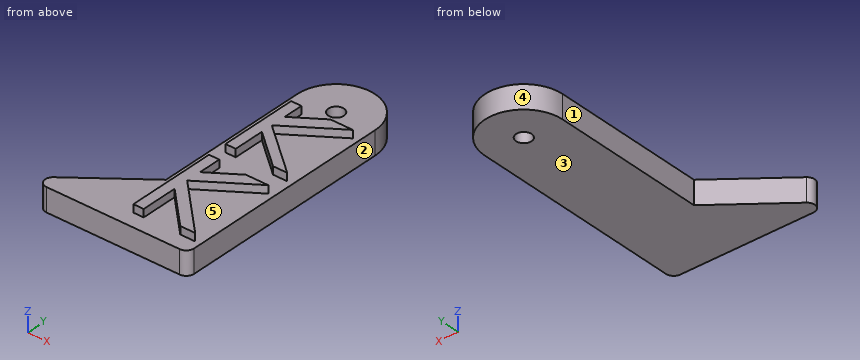
```python
from build123d import *

# Parameters (mm, degrees)
SKETCH_1_R      = 1
EXTRUDE_1_DEPTH = 3
EXTRUDE_2_DEPTH = 3
FILLET_2_R      = 1
FILLET_3_R      = 1
EXTRUDE_3_DEPTH = 1


with BuildPart() as part:
    # 草图1 → 凸台-拉伸1 (new body)
    with BuildSketch(Plane.XY):
        with BuildLine():
            Line((-5, 0), (-5, -20))
            Line((-5, -20), (5, -20))
            Line((5, -20), (5, 0))
            ThreePointArc((5, 0), (0, 5), (-5, 0))
        make_face()
        Circle(SKETCH_1_R, mode=Mode.SUBTRACT)
    extrude(amount=EXTRUDE_1_DEPTH)

    # 草图2 → 凸台-拉伸2 (add)
    with BuildSketch(Plane.XY.offset(3)):
        Polygon((5, -20), (-5, -20), (-16.053330201, -28.571505672), (5, -28.571505672), align=None)
    extrude(amount=-EXTRUDE_2_DEPTH)

    # 圆角2
    fillet_2_edges = [part.edges().sort_by_distance(p)[0] for p in [
        (-16.053330201, -28.571505672, 1.5),
    ]]
    fillet(fillet_2_edges, radius=FILLET_2_R)

    # 圆角3
    fillet_3_edges = [part.edges().sort_by_distance(p)[0] for p in [
        (5, -28.571505672, 1.5),
    ]]
    fillet(fillet_3_edges, radius=FILLET_3_R)

    # 草图3 → 凸台-拉伸3 (add)
    with BuildSketch(Plane.XY.offset(3)):
        Polygon((-3.674988176, -2.510402489), (-3.674988176, -12.516814932), (-2.349938126, -12.516814932), (-2.349938126, -8.541664784), (2.447656881, -12.516814932), (4.275312121, -12.516814932), (-2.349938126, -7.02732187), (4.275312121, -2.510402489), (1.392652218, -2.510402489), (-2.349938126, -5.062001029), (-2.349938126, -2.510402489), align=None)
        Polygon((-3.674988176, -15.023538628), (-3.674988176, -26.544068904), (-2.349938126, -26.544068904), (-2.349938126, -21.837856659), (2.356274118, -26.544068904), (4.275312121, -26.544068904), (-2.349938126, -19.918818657), (4.275312121, -15.401899276), (1.392652218, -15.401899276), (-2.349938126, -17.953497816), (-2.349938126, -15.023538628), align=None)
    extrude(amount=EXTRUDE_3_DEPTH)


solid = part.part
```
Source: CAD feature listing. Evaluate the final solid. Frame: model axes, mm. Face numbers are marked on the shaded views. A direction names the side the tool comes from. Coordinates: 2 decimals unless noted, no trailing zeros. Write each loop counter-clockwise with the first axis right and the second up, starting at its lowest first coordinate (ties: lowest second). Pieces come first, ordered by that corner, then holes. Notation, with made-up numbers: (-35, 19.5) -> (-28, 19.5) arc R27 ccw to (-28, 48.5) -> close; hole circle Ø4 at (-31, 24.25). An arc over 180 degrees is marked (long way). Return JSON: item names as keys, results as strings. Group by question number.
1) Section query D-D, the plane x = -10.25. Return loops of the section in (y, z).
2) Section query B-B, the plane x = 0. Return loops of the section in (y, z).
3) Mould query, pull axis Y, two halves, no side actions, for the marked faces 3, 4 and 5. Classes: +Y half, -Y half, draft (parallel to the pull), parting line (faces both ways), or undercut.
4) Contact query for flat-ended pins moving along their axis: P1, Ø0.5, axis at y = -9.5, z = 3.5, coming from the +X side; P2, Ø1.8, axis at x = 0, y = 0, coming from the +Z side; P3, Ø1, axis at y = -24.5, z = 2, coming from the -X side; P4, Ø0.5, axis at y = -9.5, z = 3.5, coming from the -X side (3 decimals). Output: stop coordinate, or through.
5) Ray query, line 1 along Y through (x, z) = (0, 2.35); line 2 along Y through (x, z) = (-2.5, 3.4); line 3 along X through (y, z) = (-9.5, 1.55). Return the intervals inside material, ascending.
6) Set-up query: the marked faces 1 and 2. Return all of +Z, -Z, +X, -X, +Y, -Y with unobstructed straight access to the full face (end or side cutting, diameter ignored); none if empty.
7) Section query A-A, the plane z = 0.55. Return loops of the section in (x, y).
8) Section query C-C, the plane y = -4. Return loops of the section in (x, z), plus the area to 3 significant figures.
From the geometry:
{
 "1": {"outline": "(-28.57, 0) -> (-24.07, 0) -> (-24.07, 3) -> (-28.57, 3) -> close"},
 "2": {"outline": "(-28.57, 0) -> (-1, 0) -> (-1, 3) -> (-3.46, 3) -> (-3.46, 4) -> (-5.43, 4) -> (-5.43, 3) -> (-8.97, 3) -> (-8.97, 4) -> (-10.49, 4) -> (-10.49, 3) -> (-16.35, 3) -> (-16.35, 4) -> (-18.32, 4) -> (-18.32, 3) -> (-22.27, 3) -> (-22.27, 4) -> (-24.19, 4) -> (-24.19, 3) -> (-28.57, 3) -> close; (1, 0) -> (5, 0) -> (5, 3) -> (1, 3) -> close"},
 "3": {"face 3": "draft", "face 4": "+Y half", "face 5": "undercut"},
 "4": {"P1": "x = 0.94", "P2": "through", "P3": "x = -11.45", "P4": "x = -3.675"},
 "5": {"line 1": "-28.57 to -1, 1 to 5", "line 2": "-26.54 to -15.02, -12.52 to -2.51", "line 3": "-5 to 5"},
 "6": {"face 1": "+Z, -Z, -X, +Y", "face 2": "+Z, -Z, +X, +Y, -Y"},
 "7": {"outline": "(-13.74, -26.78) arc R1 ccw to (-13.13, -28.57) -> (4, -28.57) arc R1 ccw to (5, -27.57) -> (5, 0) arc R5 ccw to (-5, 0) -> (-5, -20) -> close; hole circle Ø2 at (0, 0)"},
 "8": {"outline": "(-5, 0) -> (5, 0) -> (5, 3) -> (2.09, 3) -> (2.09, 4) -> (-0.79, 4) -> (-0.79, 3) -> (-2.35, 3) -> (-2.35, 4) -> (-3.67, 4) -> (-3.67, 3) -> (-5, 3) -> close", "area": "34.2 mm²"}
}
